Could you check a few things on this drawing? It's one solid part, dimensions in mm from its lowest x, y, z. Coordinates: 2 decimals unless noted, no trailing zeros. Write each loop counter-clockwise with the first axis right and the second up, starting at its lowest first coordinate (ties: lowest second). Pieces come first, ordered by that corner, then holes.
Item 1: Please list where these lines run through material, in increasing order: line 1 (Y direction, x = 35.25, z = 6); line 2 (X direction, y = 8.25, z = 1.5); line 3 (Z direction, x = 60, y = 9.25).
Item 2: I want a section at C-C (y = 9.5). Please give me the cut outline in (x, z), and give its area (3 significant figures).
Item 3: If we mould it in two halves opening along Y, with no side actions, what happens to the marked faces 1, 2 and 3? For each: pulls with the +Y half, pulls with the -Y half, needs draft (parallel to the pull), parting line crosses it, or undercut.
Item 4: I want a section at A-A (y = 6). Please give me the cut outline in (x, z), and give its area (3 significant figures).
Item 5: I want a section at B-B (x = 75). Please give me the cut outline in (y, z).
Item 6: I'm going to push a flat-ended pin straight in: P1, Ø1.9, axis at x = 5, z = 6, coming from the -Y side. Where does the tip first touch, or does it pass through?
Item 7: I want a section at D-D (z = 6). Please give me the cut outline in (x, y), and give its area (3 significant figures).
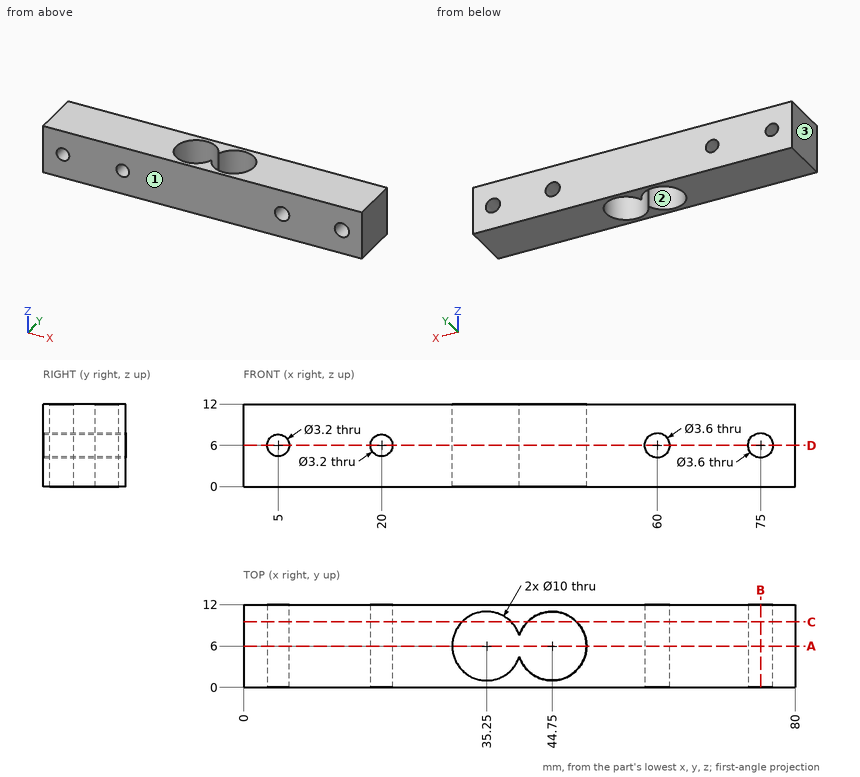
Answer:
1. line 1: y = 0 to 1, 11 to 12
1. line 2: x = 0 to 30.78, 39.72 to 40.28, 49.22 to 80
1. line 3: z = 0 to 4.2, 7.8 to 12
2. outline: (0, 0) - (31.68, 0) - (31.68, 12) - (0, 12) - close; (38.82, 0) - (41.18, 0) - (41.18, 12) - (38.82, 12) - close; (48.32, 0) - (80, 0) - (80, 12) - (48.32, 12) - close; hole circle Ø3.2 at (5, 6); hole circle Ø3.2 at (20, 6); hole circle Ø3.6 at (60, 6); hole circle Ø3.6 at (75, 6)
2. area: 752 mm2
3. face 1: pulls with the -Y half
3. face 2: undercut
3. face 3: needs draft
4. outline: (0, 0) - (30.25, 0) - (30.25, 12) - (0, 12) - close; (49.75, 0) - (80, 0) - (80, 12) - (49.75, 12) - close; hole circle Ø3.2 at (5, 6); hole circle Ø3.2 at (20, 6); hole circle Ø3.6 at (60, 6); hole circle Ø3.6 at (75, 6)
4. area: 690 mm2
5. outline: (0, 0) - (12, 0) - (12, 4.2) - (0, 4.2) - close; (0, 7.8) - (12, 7.8) - (12, 12) - (0, 12) - close
6. P1: passes through
7. outline: (0, 0) - (3.4, 0) - (3.4, 12) - (0, 12) - close; (6.6, 0) - (18.4, 0) - (18.4, 12) - (6.6, 12) - close; (21.6, 0) - (58.2, 0) - (58.2, 12) - (21.6, 12) - close; (61.8, 0) - (73.2, 0) - (73.2, 12) - (61.8, 12) - close; (76.8, 0) - (80, 0) - (80, 12) - (76.8, 12) - close; hole (40, 4.44) arc R5 ccw (long way) to (40, 7.56) arc R5 ccw (long way) to start
7. area: 641 mm2
